For this review, use the dimensioned drawing (mm, ordinates from the lowest corner) and the shaded views. Round coordinates to 2 decimals unless told otherwise and drop trailing zeros. Loops run counter-clockwise (first coordinate to the right, second up) from the corner with the lowest first, then second, coordinate; pieces in that order, holes last. Notation, with made-up numbers: (37.25, -33) -> (65.25, -33) arc R23 ccw to (65.25, -9) -> close; hole circle Ø8 at (12.25, -8.75). An arc over 180 degrees is marked (long way). Write each question's results on one line, items separated by ' | '. Start each with the question number.
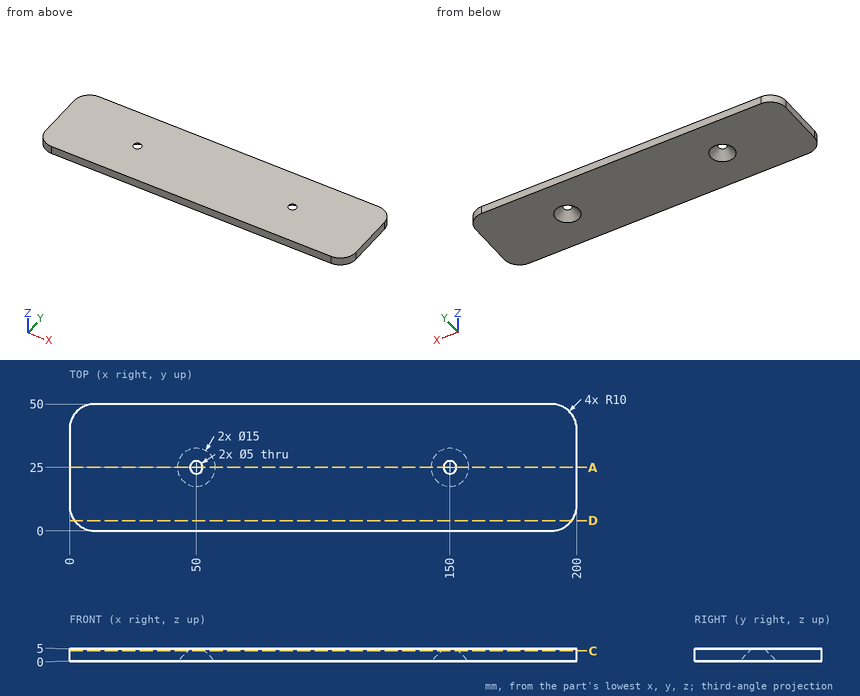
1) Take a section at A-A (y = 25). State how many separate pieces and enclosed holes the cut face has, plus the area to 3 significant figures.
2) Take a section at D-D (y = 4). Write out the cut boundary in (x, z).
3) Take a section at C-C (z = 4.15). Write out the cut boundary in (x, y).
4) To check wall thickness, follow line 1 (X direction, y = 28, z = 1.6); line 2 (X direction, y = 24.5, z = 0.7); line 3 (Y direction, x = 144.5, z = 0.65). State the ranges of each line that lie inside material, in increasing order. Write a range as from..to.
Geometry check:
1) separate pieces: 3 | enclosed holes: 0 | area: 900 mm^2
2) outline: (2, 0) -> (198, 0) -> (198, 5) -> (2, 5) -> close
3) outline: (0, 10) arc R10 ccw to (10, 0) -> (190, 0) arc R10 ccw to (200, 10) -> (200, 40) arc R10 ccw to (190, 50) -> (10, 50) arc R10 ccw to (0, 40) -> close; hole circle Ø6.7 at (50, 25); hole circle Ø6.7 at (150, 25)
4) line 1: x = 0..44.92, 55.08..144.92, 155.08..200 | line 2: x = 0..43.22, 56.78..143.22, 156.78..200 | line 3: y = 0..20.92, 29.08..50
